Part print with two shaded views. Sizes in mm from the minimum x, y, z corner. Round coordinates to 2 decimals unless told otherwise and drop trailing zeros. Write each loop counter-clockwise with the first axis right and the second up, starting at its lowest first coordinate (ties: lowest second). Pieces come first, ordered by that corner, then holes.
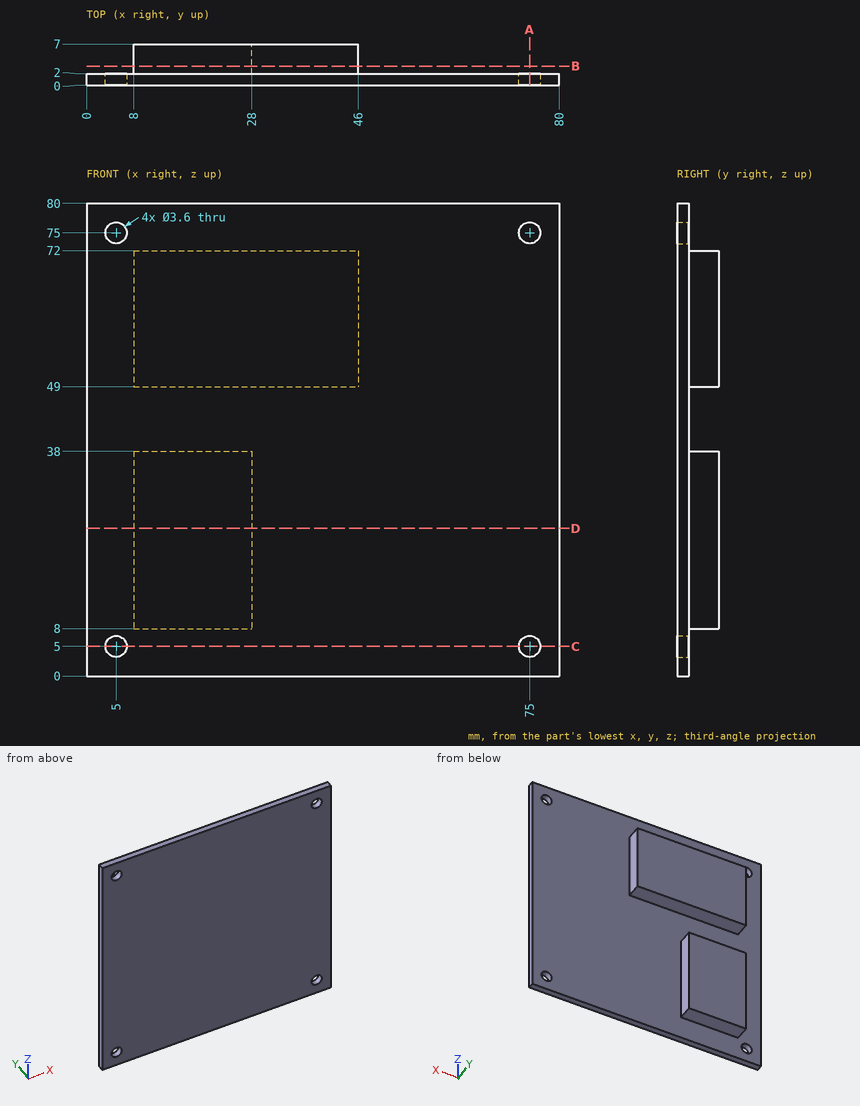
Q1. Cut at B-B on y = 3.25. Write the cut outline in (x, z), plus the area to 3 significant figures.
Values follow:
outline: (8, 8) - (28, 8) - (28, 38) - (8, 38) - close; (8, 49) - (46, 49) - (46, 72) - (8, 72) - close
area: 1,470 mm2
Q2. Cut at D-D on z = 25. Write the cut outline in (x, y).
Values follow:
outline: (0, 0) - (80, 0) - (80, 2) - (28, 2) - (28, 7) - (8, 7) - (8, 2) - (0, 2) - close
Q3. Cut at C-C on z = 5. Write the cut outline in (x, y), plus the area to 3 significant figures.
Values follow:
outline: (0, 0) - (3.2, 0) - (3.2, 2) - (0, 2) - close; (6.8, 0) - (73.2, 0) - (73.2, 2) - (6.8, 2) - close; (76.8, 0) - (80, 0) - (80, 2) - (76.8, 2) - close
area: 146 mm2
Q4. Drop flat-ended pins along their axis: pin 1 (4 mm diameter, centred on x = 75, z = 75, fed in from +Y); pin 2 (2.5 mm diameter, centred on x = 33, y = 4.5, fed in from -Z); pin 3 (1.5 mm diameter, centred on y = 4, z = 62.5, fed in from +X). Give the stop position or say it passes through.
Values follow:
pin 1: stops at y = 2
pin 2: stops at z = 49
pin 3: stops at x = 46
Q5. Cut at A-A on x = 75. Write the cut outline in (y, z), plus the area to 3 significant figures.
Values follow:
outline: (0, 0) - (2, 0) - (2, 3.2) - (0, 3.2) - close; (0, 6.8) - (2, 6.8) - (2, 73.2) - (0, 73.2) - close; (0, 76.8) - (2, 76.8) - (2, 80) - (0, 80) - close
area: 146 mm2
Q6. Wall check: L1, parallel to Z at x = 5, y = 0.75; L2, parallel to Z at x = 10.5, y = 3.25. Give the ranges that are in metal, low to high.
Values follow:
L1: z = 0 to 3.2, 6.8 to 73.2, 76.8 to 80
L2: z = 8 to 38, 49 to 72
